Autodesk Inventor part; units mm, degrees
ref_plane "b600_1_XY" through (8.5, 0, 0) normal (1, 0, 0) x (0, 0, -1)
ref_plane "b600_1_YZ" through (8.5, 0, 0) normal (0, 0, -1) x (0, 1, 0)
ref_plane "b600_1_ZX" through (8.5, 0, 0) normal (0, 1, 0) x (1, 0, 0)
sketch "_____2" plane through (0, 0, 0) normal (0, 0, 1) x (1, 0, 0)
  line L0 (11, 0) -> (-11, 0)
  line L1 (-11, 0) -> (-11, 10)
  line L2 (-11, 10) -> (-9.5, 10)
  line L3 (-9.5, 10) -> (-9.5, 12.3683)
  line L4 (-9.5, 12.3683) -> (-10.4037, 15.7412)
  line L5 (-10.4037, 15.7412) -> (-9.4378, 16)
  line L6 (-9.4378, 16) -> (-8.5, 12.5)
  line L7 (-8.5, 12.5) -> (8.5, 12.5)
  line L8 (8.5, 12.5) -> (9.4378, 16)
  line L9 (9.4378, 16) -> (10.4037, 15.7412)
  line L10 (10.4037, 15.7412) -> (9.5, 12.3683)
  line L11 (9.5, 12.3683) -> (9.5, 10)
  line L12 (9.5, 10) -> (11, 10)
  line L13 (11, 10) -> (11, 0)
  line L14 (11, 0) -> (-11, 0)
revolve "Revolution1" add sketch "_____2" angle 360 about axis through (11, 0, 0) along (1, 0, 0)
sketch "_____3" plane through (0, 0, 0) normal (0, 0, 1) x (1, 0, 0)
  line L0 (11, 0) -> (-11, 0)
  line L1 (-11, 0) -> (-11, 8)
  line L2 (-11, 8) -> (-6, 8)
  line L3 (-6, 8) -> (-6, 7)
  line L4 (-6, 7) -> (6, 7)
  line L5 (6, 7) -> (6, 8)
  line L6 (6, 8) -> (11, 8)
  line L7 (11, 8) -> (11, 0)
  line L8 (11, 0) -> (-11, 0)
revolve "Revolution2" cut sketch "_____3" angle 360 about axis through (11, 0, 0) along (1, 0, 0)
ref_plane "b600_1_XY" through (8.5, 0, 0) normal (1, 0, 0) x (0, 0, -1)
ref_plane "b600_1_YZ" through (8.5, 0, 0) normal (0, 0, -1) x (0, 1, 0)
ref_plane "b600_1_ZX" through (8.5, 0, 0) normal (0, 1, 0) x (1, 0, 0)
ref_plane "b600_2_XY" through (-8.5, 0, 0) normal (1, 0, 0) x (0, 0, -1)
ref_plane "b600_2_YZ" through (-8.5, 0, 0) normal (0, 0, -1) x (0, 1, 0)
ref_plane "b600_2_ZX" through (-8.5, 0, 0) normal (0, 1, 0) x (1, 0, 0)
ref_plane "to_dummy_XY" through (0, 0, 0) normal (1, 0, 0) x (0, 0, -1)
ref_plane "to_dummy_YZ" through (0, 0, 0) normal (0, 0, -1) x (0, 1, 0)
ref_plane "to_dummy_ZX" through (0, 0, 0) normal (0, 1, 0) x (1, 0, 0)
properties part number "C-AFDF22-25_bw"
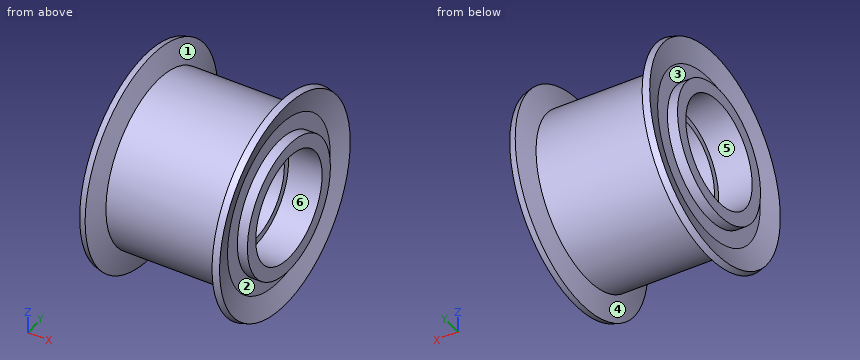
The listing builds one solid part. Answer for the finished solid, in the listing's coordinates (mm). Face numbers are marked on the shaded views. A direction names the side the tool comes from. Give positions to 0.01 mm unless a question says otherwise; leave off trailing zeros. Loops run counter-clockwise (first coordinate to the right, second up) from the corner with the lowest first, then second, coordinate; pieces in that order, holes last.
Item 1: Find the intervals of material crossed by line 1 along Z through (x, y) = (1.25, 0); line 2 along X through (y, z) = (-4.5, 9.5); line 3 along X through (y, z) = (10, 8.5), in increasing order.
Derived:
line 1: z = -12.5 to -7, 7 to 12.5
line 2: x = -9.5 to 9.5
line 3: x = -9.7 to -8.67, 8.67 to 9.7
Item 2: A tool of negligible diameter and unlimited length cuts with its end or side. For the marked faces 1, 2 and 3, from which of +Z, -Z, +X, -X, +Y, -Y can it reach the whole face along a straight path? Write none if from no direction.
Derived:
face 1: none
face 2: +X
face 3: -X
Item 3: A cutting plane is placed at A-A (x = 2). Give the vertices of the cut face in (y, z), then the cut area to 3 significant figures.
Derived:
outline: circle Ø25 at (0, 0); hole circle Ø14 at (0, 0)
area: 337 mm2
Item 4: Determine the mould class of the marked faces 4, 5 and 6 for opening direction Y: +Y half, -Y half, draft (parallel to the pull), parting line (faces both ways), or undercut.
Derived:
face 4: parting line
face 5: undercut
face 6: undercut
Item 5: Each of these flat-tipped pins is pushed along its axis until it touches: pin 1 Ø2 at (x, z) = (-6, -4.5) entering from +Y; pin 2 Ø14.5 at (y, z) = (0, 0) entering from +X; pin 3 Ø3 at (x, z) = (-3, 1) entering from +Y. Where does it stop, or does it pass through?
Derived:
pin 1: stops at y = 12
pin 2: stops at x = 6
pin 3: stops at y = 12.5
